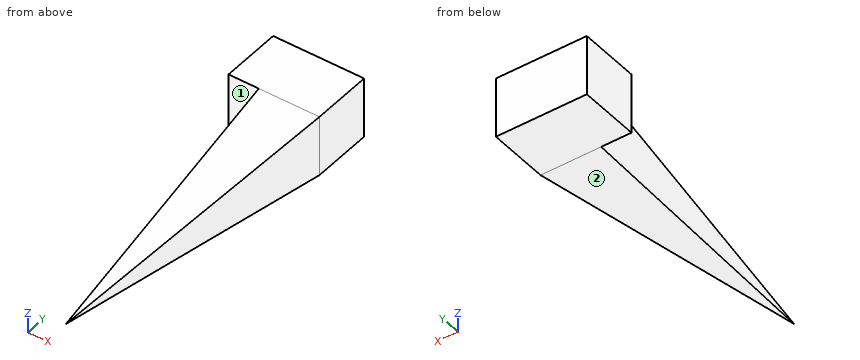
```python
from build123d import *

# Parameters (mm, degrees)
F0_W     = 10
F0_H     = 50
F0_H_2   = 10
F0_W_2   = 5
F1_DEPTH = 10
F2_SIZE2 = 49.99999
F2_SIZE  = 4.99999


# Not quite as in the source:
# - a fillet or chamfer is up to 0.001 mm smaller than in the source, because OpenCascade refuses the exact size


with BuildPart() as f1:
    # F0 (on Top) → F1 (new body)
    with BuildSketch(Plane.XY):
        with Locations((-5, -25)):
            Rectangle(F0_W, F0_H)
        with Locations((-5, 5)):
            Rectangle(F0_W, F0_H_2)
        with Locations((-12.5, 5)):
            Rectangle(F0_W_2, F0_H_2)
    extrude(amount=F1_DEPTH)

    # F2 (size 5 and 50 in the source; OpenCascade refuses exactly that, so slightly less here)
    f2_edges = [f1.edges().sort_by_distance(p)[0] for p in [
        (-5, -50, 10),
        (-10, -50, 5),
        (-5, -50, 0),
        (0, -50, 5),
    ]]
    f2_side = f1.faces().sort_by_distance((-5, -50, 5))[0]
    chamfer(f2_edges, length=F2_SIZE, length2=F2_SIZE2, reference=f2_side)


solid = f1.part
```
CAD build for the part. Positions are in the model's coordinates, mm. Face numbers are marked on the shaded views. A direction names the side the tool comes from. Give positions to 0.01 mm unless a question says otherwise; leave off trailing zeros. Order: outer loops, then holes, each group sorted by start corner. A loop starts at its lowest first (then second) coordinate and runs counter-clockwise, first axis right, second up.
(1) Tool access for the marked faces 1 and 2: list every direction of +Z, -Z, +X, -X, +Y, -Y with a clear straight run to the whole face (end or side of a thin tool).
(2) Drill centre lines: L1, parallel to Y at x = -14, z = 0.5; L2, parallel to Z at x = -6, y = -28.5; L3, parallel to Z at x = -4.5, y = -42.5. Where is each one in solid material? Low to high.
(3) Saw through at B-B, the plane y = -29. Give the cut face in (x, z).
(4) Saw through at C-C, the plane x = -6.75. Give the cut face in (y, z), then the cut area to 3 significant figures.
(5) Flat gauge pins, fed straight in: pin 1 (6 mm diameter, centred on x = -8, y = -39, fed in from -Z); pin 2 (8 mm diameter, centred on x = -4, y = -20.5, fed in from -Z). Where does each tip first touch, or does it go through?
Results found:
1. face 1: +Z, -Z, -X, -Y
1. face 2: -Z, +X, -X, -Y
2. L1: y = 0 to 10
2. L2: z = 2.85 to 7.15
2. L3: z = 4.25 to 5.75
3. outline: (-7.1, 2.9) - (-2.9, 2.9) - (-2.9, 7.1) - (-7.1, 7.1) - close
4. outline: (-32.5, 3.25) - (0, 0) - (10, 0) - (10, 10) - (0, 10) - (-32.5, 6.75) - close
4. area: 319 mm2
5. pin 1: stops at z = 3.65
5. pin 2: stops at z = 1.65
